For this review, take the finished solid that the model builds, in its own axes (mm). Coordinates: 2 decimals unless noted, no trailing zeros. Write each loop counter-clockwise with the first axis right and the second up, starting at its lowest first coordinate (ties: lowest second). Pieces come first, ordered by that corner, then holes. Notation, with made-up numbers: M 10,19.5 L 66,19.5 A20 ccw 66,49.5 Z; hole C 33,53.25 d7. An arc over 180 degrees is marked long. Return JSON: item names as keys, results as strings.
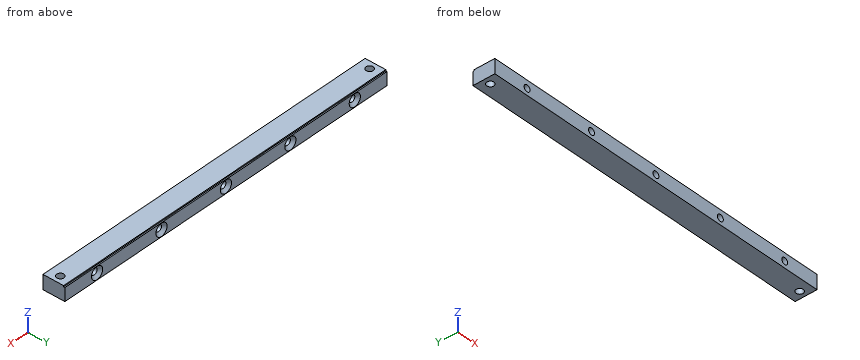
```python
from build123d import *

# Parameters (mm, degrees)
SKETCH_1_W                 = 300
SKETCH_1_H                 = 12
EXTRUDE_275_DEPTH          = 18.35
SKETCH_2_W                 = 300
SKETCH_2_H                 = 1
CUT_EXTRUDE_1_DEPTH        = 1
HOLE_WIZARD_M4_D           = 5.5
HOLE_WIZARD_M4_CSINK_D     = 10.4
HOLE_WIZARD_M4_CSINK_ANGLE = 90
PATTERN_LINEAR_1_COUNT     = 3
PATTERN_LINEAR_1_PITCH     = 60
PATTERN_LINEAR_1_COL_COUNT = 3
PATTERN_LINEAR_1_COL_PITCH = 60
SKETCH_5_R                 = 3
CUT_EXTRUDE_6_DEPTH        = 152.593939523


with BuildPart() as part:
    # Эскиз1 → Extrude 275 (new body)
    with BuildSketch(Plane(origin=(0, 0, 0), x_dir=(1, 0, 0), z_dir=(0, 1, 0))):
        with Locations((0, 6)):
            Rectangle(SKETCH_1_W, SKETCH_1_H)
    extrude(amount=EXTRUDE_275_DEPTH)

    # Эскиз2 → Вырез-Вытянуть1 (cut)
    with BuildSketch(Plane(origin=(0, 18.35, 0), x_dir=(1, 0, 0), z_dir=(0, 1, 0))):
        with Locations((0, 0.5)):
            Rectangle(SKETCH_2_W, SKETCH_2_H)
    extrude(amount=-CUT_EXTRUDE_1_DEPTH, mode=Mode.SUBTRACT)

    # Крепление-M4 (through all)
    with Locations(Plane(origin=(0, 18.35, 0), x_dir=(-1, 0, 0), z_dir=(0, 1, 0))):
        with Locations((0, -6.5)):
            hole_wizard_m4 = CounterSinkHole(HOLE_WIZARD_M4_D / 2, HOLE_WIZARD_M4_CSINK_D / 2, counter_sink_angle=HOLE_WIZARD_M4_CSINK_ANGLE)

    # Линейный массив1: Крепление-M4 ×3
    with Locations(*[(-i * PATTERN_LINEAR_1_PITCH, 0, 0) for i in range(1, PATTERN_LINEAR_1_COUNT)]):
        add(hole_wizard_m4, mode=Mode.SUBTRACT)

    # Линейный массив1 col: Крепление-M4 ×3
    with Locations(*[(i * PATTERN_LINEAR_1_COL_PITCH, 0, 0) for i in range(1, PATTERN_LINEAR_1_COL_COUNT)]):
        add(hole_wizard_m4, mode=Mode.SUBTRACT)

    # Эскиз5 → Валы-6мм (cut, through all)
    with BuildSketch(Plane.XY.offset(-12)):
        with Locations((-144, 9.175)):
            Circle(SKETCH_5_R)
        with Locations((144, 9.175)):
            Circle(SKETCH_5_R)
    extrude(amount=CUT_EXTRUDE_6_DEPTH, mode=Mode.SUBTRACT)


solid = part.part
```
1. Wall thickness on L1, parallel to Z at x = -120.5, y = 6.5; L2, parallel to Y at x = 144, z = -3 (3 decimals); L3, parallel to X at y = 15.5, z = -9: over which ranges is each line inside the solid? List them lowest first. Write a range as from..to.
Checks:
{"L1": "-12..-9.2, -3.8..0", "L2": "0..6.175, 12.175..18.35", "L3": "-150..-121.15, -118.85..-61.15, -58.85..-1.15, 1.15..58.85, 61.15..118.85, 121.15..150"}
2. Clearance check with flat-ended pins moving along their axes: pin 1 Ø4.5 at (x, z) = (0, -6.5) entering from +Y; pin 2 Ø0.8 at (x, z) = (28.5, -0.5) entering from +Y. State where each tip first meets the part, or that it passes through.
Checks:
{"pin 1": "through", "pin 2": "y = 17.35"}
3. We need section B-B (x = -60). State the section outline as (y, z) points, plus the area to 3 significant figures.
Checks:
{"outline": "M 0,-12 L 18.35,-12 L 18.35,-11.7 L 15.9,-9.25 L 0,-9.25 Z; M 0,-3.75 L 15.9,-3.75 L 18.35,-1.3 L 18.35,-1 L 17.35,-1 L 17.35,0 L 0,0 Z", "area": "112 mm2"}
4. We need section A-A (x = -144). State the section outline as (y, z) points (3 decimals), plus the area to 3 significant figures.
Checks:
{"outline": "M 0,-12 L 6.175,-12 L 6.175,0 L 0,0 Z; M 12.175,-12 L 18.35,-12 L 18.35,-1 L 17.35,-1 L 17.35,0 L 12.175,0 Z", "area": "147 mm2"}
